For this review, use the dimensioned drawing (mm, ordinates from the lowest corner) and the shaded views. Coordinates: 2 decimals unless noted, no trailing zeros. Write each loop counter-clockwise with the first axis right and the second up, starting at its lowest first coordinate (ties: lowest second). Pieces come first, ordered by that corner, then holes. Notation, with made-up numbers: (-5.5, -28.5) - (34.5, -28.5) arc R19 cw to (34.5, -16.5) - close; hole circle Ø7 at (30.5, 10.25). An arc over 180 degrees is marked (long way). One line per item, written item: value.
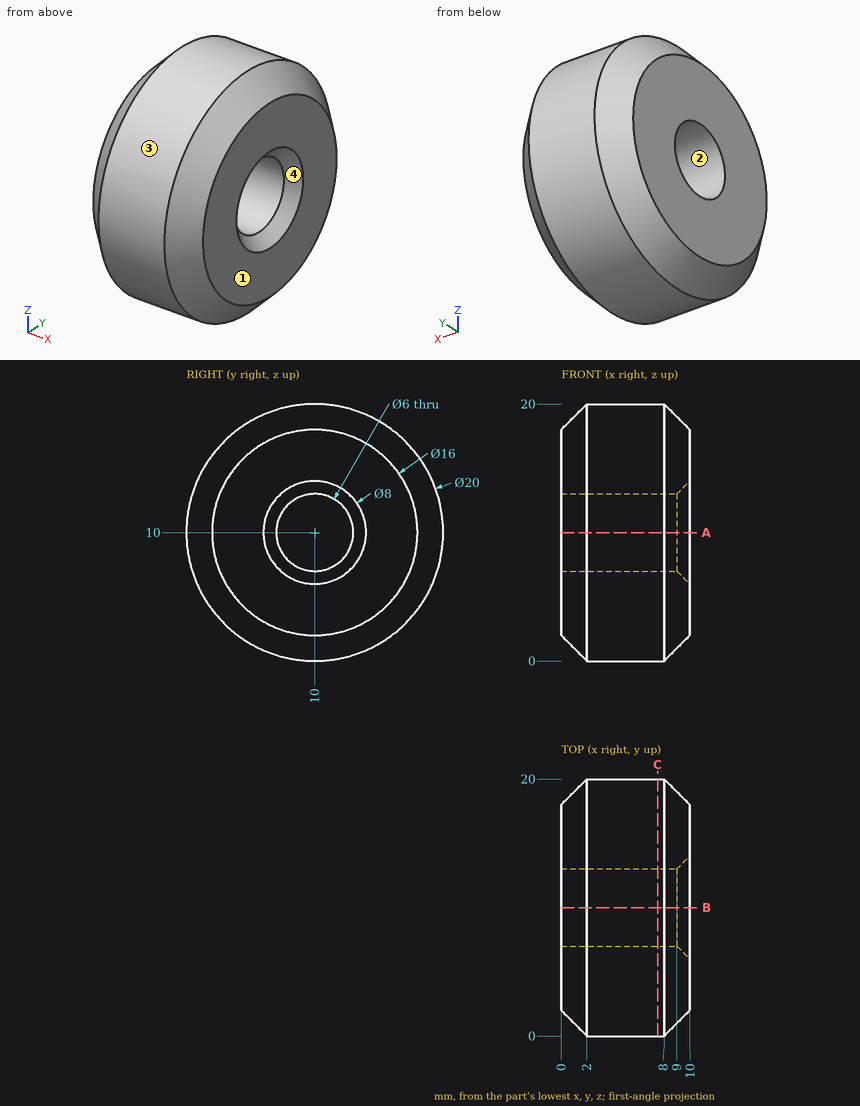
1. Consider section A-A, the plane z = 10. Write out the cut boundary in (x, y), then the cut area to 3 significant figures.
Answer block:
outline: (0, 2) - (2, 0) - (8, 0) - (10, 2) - (10, 6) - (9, 7) - (0, 7) - close; (0, 13) - (9, 13) - (10, 14) - (10, 18) - (8, 20) - (2, 20) - (0, 18) - close
area: 131 mm^2
2. Mouldability with a two-part tool opening along Z and no side actions: class the marked faces 1, 2, 3 and 4 as released by +Z, released by -Z, zero draft, split by the parting line, or undercut.
Answer block:
face 1: zero draft
face 2: undercut
face 3: split by the parting line
face 4: undercut
3. Insertion check: pin 1 Ø6 at (x, y) = (3.5, 17.5) entering from +Z; pin 2 Ø1 at (x, y) = (2, 3.5) entering from +Z; pin 3 Ø3 at (x, y) = (2, 12) entering from +Z. Each pin has a flat end and moves straight along its axis. Give the tip position at first contact, or say it passes through.
Answer block:
pin 1: stops at z = 18.93
pin 2: stops at z = 18
pin 3: stops at z = 19.99
4. Wall thickness on line 1 along Z through (x, y) = (5.25, 10); line 2 along Y through (x, z) = (7.75, 11.25); line 3 along Y through (x, z) = (3.75, 9.75): over which ranges is each line inside the solid? List them lowest first.
Answer block:
line 1: z = 0 to 7, 13 to 20
line 2: y = 0.08 to 7.27, 12.73 to 19.92
line 3: y = 0 to 7.01, 12.99 to 20
5. Consider section C-C, the plane x = 7.5. Write out the cut boundary in (y, z), then the cut area to 3 significant figures.
Answer block:
outline: circle Ø20 at (10, 10); hole circle Ø6 at (10, 10)
area: 286 mm^2
